Design review of the part built by this model. Coordinates are the model's own, in mm. A direction names the side the tool comes from. Give positions to 0.01 mm unless a question says otherwise; leave off trailing zeros. Write each loop counter-clockwise with the first axis right and the second up, starting at its lowest first coordinate (ties: lowest second). Pieces come first, ordered by that corner, then holes. Notation, with made-up numbers: (-36.5, 77.5) - (6.5, 77.5) arc R34 cw to (6.5, 113.5) - close; hole circle Ø1 at (49, -9.5). An arc over 180 degrees is marked (long way). Use a Markdown table: item, result. Add a question column.
Autodesk Inventor part; units mm, degrees
ref_plane "YZ Plane" through (0, 0, 0) normal (1, 0, 0) x (0, 1, 0)
ref_plane "XZ Plane" through (0, 0, 0) normal (0, 1, 0) x (-1, 0, 0)
ref_plane "XY Plane" through (0, 0, 0) normal (0, 0, 1) x (1, 0, 0)
sketch "Sketch1" plane through (0, 0, 0) normal (1, 0, 0) x (0, 1, 0)
  circle A0 centre (0, 0) radius 20.5
  circle A1 centre (0, 0) radius 15 construction
  line L0 (0, 0) -> (16.0369, -27.7767) construction
  line L1 (16.0369, -27.7767) -> (16.0369, 0) construction
  line L2 (16.0369, 0) -> (0, 0) construction
  circle A2 centre (0, 0) radius 14.25 construction
  line L3 (0, 0) -> (-15.2425, -26.4009) construction
  line L4 (-15.2425, -26.4009) -> (-20.5, 0) construction
  line L5 (0, 0) -> (-20.5, 0) construction
  circle A3 centre (7.5, -12.9904) radius 2
  circle A4 centre (7.5, 12.9904) radius 2
  circle A5 centre (-15, 0) radius 2
  circle A6 centre (14.25, 0) radius 2
  circle A7 centre (-7.125, 12.3409) radius 2
  circle A8 centre (-7.125, -12.3409) radius 2
  dimension "d0" = 41
  dimension "d1" = 30
  dimension "d16" = 28.5
  dimension "d15" = 60
  dimension "d22" = 60
  dimension "d28" = 4
  dimension "d31" = 360
  dimension "d33" = 4
  dimension "d36" = 360
extrude "Extrusion1" add sketch "Sketch1" along normal blind 3
chamfer "Chamfer2" distance 0.5 angle 45 1 edges at (0, -20.5, 0)
chamfer "Chamfer3" distance 2 angle 45 3 edges at (3, 5.5, -12.9904) (3, -17, 0) (3, 5.5, 12.9904)
sketch "Sketch5" plane through (3, 0, 0) normal (1, 0, 0) x (0, 0, -1)
  circle A0 centre (0, 0) radius 5
  dimension "d44" = 10
extrude "Extrusion3" add sketch "Sketch5" along normal blind 8
sketch "Sketch6" plane through (11, 0, 0) normal (1, 0, 0) x (0, 0, -1)
  line L0 (-1, 4) -> (-1, 6)
  line L1 (-1, 6) -> (1, 6)
  line L2 (1, 6) -> (1, 4)
  line L3 (1, 4) -> (-1, 4)
  circle A0 centre (0, 0) radius 5
  line L4 (-1, 4) -> (1, 6) construction
  line L5 (-1, 6) -> (1, 4) construction
  point P0 (0, 5)
  point P1 (-1, 4.899)
  point P2 (1, 4.899)
  dimension "d47" = 2
  dimension "d48" = 2
extrude "Extrusion4" add sketch "Sketch6" against normal blind 8 contours L0 L1 L2 A0
sketch "Sketch7" plane through (11, 0, 0) normal (1, 0, 0) x (0, 0, -1)
  circle A0 centre (0, 0) radius 2
  dimension "d51" = 4
extrude "Extrusion5" cut sketch "Sketch7" against normal blind 10.4
properties part number "small_gear_connector"
(1) Add section D-D (y = -7.5). Count the separate pieces of the cut face and the enclosed holes in it, and give its area (3 significant figures).
(2) Mouldability with a two-part tool opening along Z and no side actions: class faces 4 (the face through (6, -2, 0)), 5 (the face through (0.493, 7.24, -14.973)), 6 (the face through (7.1, 5.5, -1)), 7 (the face through (7, 6, 0)) as +Z half, -Z half, draft (parallel to the pull), parting line (faces both ways), or undercut.
(3) Add section B-B (x = 5). State the section outline as (y, z) points, and give its area (3 significant figures).
(4) For line 1 along Y through (x, z) = (5.75, 0); line 2 along Z through (x, y) = (0.75, 7); line 3 along X through (y, z) = (-2, -5), list the stretches that pass through material, from the lowest coordinate up.
(5) Add section A-A (z = 0). State the section outline as (x, y) points, and give its area (3 significant figures).
(6) Tool access review of faces 1 (the face through (11, 2, -1)), 2 (the face through (7, -5, 0)), 3 (the face through (7.1, 5.4, 1)): name each direction out of +Z, -Z, +X, -X, +Y, -Y from which nothing blocks a thin tool from reaching the whole face with its end or side.
(7) Add section C-C (x = 1.5). State the section outline as (y, z) points (3 decimals).
(8) Insertion check: pin 1 (0.9 mm diameter, centred on x = 6.5, y = 5.5, fed in from +Z); pin 2 (5 mm diameter, centred on y = -7.12, z = 12.34, fed in from +X); pin 3 (5 mm diameter, centred on x = 3, z = 11.5, fed in from -Y). Each pin has a flat end and moves straight along its axis. Give the tip position at first contact, or say it passes through.
Answers follow:
| question | item | result |
|---|---|---|
| 1 | separate pieces | 3 |
| 1 | enclosed holes | 0 |
| 1 | area | 90.6 mm^2 |
| 2 | face 4 | undercut |
| 2 | face 5 | undercut |
| 2 | face 6 | -Z half |
| 2 | face 7 | draft |
| 3 | outline | (4.9, -1) - (6, -1) - (6, 1) - (4.9, 1) arc R5 ccw (long way) to start; hole circle Ø4 at (0, 0) |
| 3 | area | 68.0 mm^2 |
| 4 | line 1 | -5 to -2, 2 to 6 |
| 4 | line 2 | -19.27 to -14.93, -11.05 to 11.05, 14.93 to 19.27 |
| 4 | line 3 | 0 to 3 |
| 5 | outline | (0, -20) - (0.5, -20.5) - (3, -20.5) - (3, -19) - (1, -17) - (0, -17) - close; (0, -13) - (1, -13) - (3, -11) - (3, -5) - (11, -5) - (11, -2) - (0.6, -2) - (0.6, 2) - (11, 2) - (11, 6) - (3, 6) - (3, 12.25) - (0, 12.25) - close; (0, 16.25) - (3, 16.25) - (3, 20.5) - (0.5, 20.5) - (0, 20) - close |
| 5 | area | 141 mm^2 |
| 6 | face 1 | +Z, -Z, +X, +Y, -Y |
| 6 | face 2 | +X |
| 6 | face 3 | +Z, +X, +Y |
| 7 | outline | circle Ø41 at (0, 0); hole circle Ø5 at (-15, 0); hole circle Ø4 at (-7.125, -12.341); hole circle Ø4 at (-7.125, 12.341); hole circle Ø4 at (0, 0); hole circle Ø5 at (7.5, -12.99); hole circle Ø5 at (7.5, 12.99); hole circle Ø4 at (14.25, 0) |
| 8 | pin 1 | z = 1 |
| 8 | pin 2 | x = 3 |
| 8 | pin 3 | y = -18.42 |
